Input: part model. Units: mm. Frame: model coordinates. Round coordinates to 2 decimals unless told otherwise and drop trailing zeros. Loops run counter-clockwise (first coordinate to the right, second up) from the corner with the lowest first, then second, coordinate; pieces in that order, holes last. Notation, with made-up numbers: (-11, 30.25) -> (25, 30.25) arc R19 ccw to (25, 51.25) -> close; hole circle Ø2 at (39.5, -36). An arc over 180 degrees is marked (long way). Answer in a Markdown table with one row per item. Add a question column.
Q1. Pin query (flat end, axial travel): pin 1 (2.5 mm diameter, centred on y = 2.5, z = 40.5, fed in from +X); pin 2 (1 mm diameter, centred on x = 11.5, y = 4, fed in from +Z); pin 3 (1 mm diameter, centred on x = -21, y = 4, fed in from +Z). Return the tip coordinate at first contact, or that it passes through.
Q2. Section C-C, the plane z = -30. Output: boundary loops of the cut face in (x, y).
Q3. Section A-A, the plane z = -63. Output: boundary loops of the cut face in (x, y).
Q4. Section B-B, the plane x = 40.5. Output: boundary loops of the cut face in (y, z).
Q5. Section D-D, the plane y = 1.2. Give the number of separate pieces and of enclosed holes in the cut face, and give its area (3 significant figures).
Q6. Ray query, L1, parallel to X at y = 4, z = -2; L2, parallel to Z at x = 66, y = 1.6; L3, parallel to Z at x = -39, y = 0.5. Return the intervals inside material, ascending. Write a range as from..to.
```python
from build123d import *

# Parameters (mm, degrees)
SKETCH1_R                = 95.25
SKETCH1_R_2              = 88.9
BOSS_EXTRUDE1_DEPTH      = 4.699
BOSS_EXTRUDE2_DEPTH      = 4.699
SKETCH3_R                = 12.7
BOSS_EXTRUDE3_DEPTH      = 4.699
BOSS_EXTRUDE4_DEPTH      = 4.699
FILLET1_R                = 3.175
CIRPATTERN1_COUNT        = 3
FILLET1_OF_CIRPATTERN1_R = 3.175
FILLET2_R                = 1.5875


with BuildPart() as part:
    # Sketch1 → Boss-Extrude1 (new body)
    with BuildSketch(Plane(origin=(0, 0, 0), x_dir=(1, 0, 0), z_dir=(0, 1, 0))):
        with Locations(Location((0, 0, 0), (0, 0, 270))):
            Circle(SKETCH1_R)
        with Locations(Location((0, 0, 0), (0, 0, 270))):
            Circle(SKETCH1_R_2, mode=Mode.SUBTRACT)
    extrude(amount=BOSS_EXTRUDE1_DEPTH)

    # Sketch2 → Boss-Extrude2 (add)
    with BuildSketch(Plane.XZ):
        with BuildLine():
            ThreePointArc((14.09030245, 107.026472785), (0, 107.95), (-14.09030245, 107.026472785))
            Line((-14.09030245, 107.026472785), (-12.432619809, 94.435123046))
            ThreePointArc((-12.432619809, 94.435123046), (0, 95.25), (12.432619809, 94.435123046))
            Line((12.432619809, 94.435123046), (14.09030245, 107.026472785))
        make_face()
        with BuildLine():
            Line((-15.09408047, -74.690084581), (-17.609760548, -87.138432012))
            ThreePointArc((-17.609760548, -87.138432012), (0, -88.9), (17.609760548, -87.138432012))
            Line((17.609760548, -87.138432012), (15.09408047, -74.690084581))
            ThreePointArc((15.09408047, -74.690084581), (0, -76.2), (-15.09408047, -74.690084581))
        make_face()
    extrude(amount=-BOSS_EXTRUDE2_DEPTH)



with BuildPart() as body_2:
    # Sketch3 → Boss-Extrude3 (new body)
    with BuildSketch(Plane.XZ):
        with Locations(Location((0, 0, 0), (0, 0, 270))):
            Circle(SKETCH3_R)
        Polygon((0, 5.499261314), (-4.7625, 2.749630657), (-4.7625, -2.749630657), (0, -5.499261314), (4.7625, -2.749630657), (4.7625, 2.749630657), align=None, mode=Mode.SUBTRACT)
    extrude(amount=-BOSS_EXTRUDE3_DEPTH)


with BuildPart() as part_1:
    add(part.part)

    add(body_2.part)  # Boss-Extrude4 merges body 2
    # Sketch4 → Boss-Extrude4 (add)
    with BuildSketch(Plane(origin=(0, 0, 0), x_dir=(-1, 0, 0), z_dir=(0, -1, 0))):
        with BuildLine():
            Line((3.175, -88.843285481), (3.175, -12.296722124))
            ThreePointArc((3.175, -12.296722124), (0, -12.7), (-3.175, -12.296722124))
            Line((-3.175, -12.296722124), (-3.175, -88.843285481))
            ThreePointArc((-3.175, -88.843285481), (0, -88.9), (3.175, -88.843285481))
        make_face()
    boss_extrude4 = extrude(amount=-BOSS_EXTRUDE4_DEPTH)

    # Fillet1
    fillet1_edges = [part_1.edges().sort_by_distance(p)[0] for p in [
        (-3.175, 2.3495, 12.296722124),
        (3.175, 2.3495, 12.296722124),
        (3.175, 2.3495, 88.843285481),
        (-3.175, 2.3495, 88.843285481),
    ]]
    fillet(fillet1_edges, radius=FILLET1_R)

    # CirPattern1: Boss-Extrude4 ×3 about axis
    cirpattern1_axis = Axis((0, 0, 0), (0, 1, 0))
    for i in range(1, CIRPATTERN1_COUNT):
        add(boss_extrude4.rotate(cirpattern1_axis, i * 360 / CIRPATTERN1_COUNT))

    # Fillet1 of CirPattern1
    fillet1_of_cirpattern1_edges = [part_1.edges().sort_by_distance(p)[0] for p in [
        (12.236773743, 2.3495, -3.398730405),
        (9.061773743, 2.3495, -8.897991719),
        (75.353042182, 2.3495, -47.171273397),
        (78.528042182, 2.3495, -41.672012083),
        (-9.061773743, 2.3495, -8.897991719),
        (-12.236773743, 2.3495, -3.398730405),
        (-78.528042182, 2.3495, -41.672012083),
        (-75.353042182, 2.3495, -47.171273397),
    ]]
    fillet(fillet1_of_cirpattern1_edges, radius=FILLET1_OF_CIRPATTERN1_R)

    # Fillet2
    fillet2_edges = [part_1.edges().sort_by_distance(p)[0] for p in [
        (-15.09408047, 2.3495, -74.690084581),
        (15.09408047, 2.3495, -74.690084581),
        (17.609760548, 2.3495, -87.138432012),
        (-17.609760548, 2.3495, -87.138432012),
        (-12.432619809, 2.3495, 94.435123046),
        (12.432619809, 2.3495, 94.435123046),
    ]]
    fillet(fillet2_edges, radius=FILLET2_R)


solid = part_1.part
```
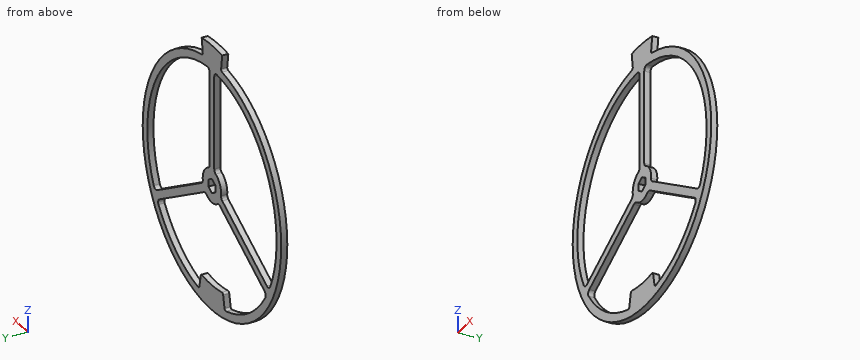
Answer block:
| question | item | result |
|---|---|---|
| 1 | pin 1 | x = 86.79 |
| 1 | pin 2 | z = 107.39 |
| 1 | pin 3 | z = 93.02 |
| 2 | outline | (-90.4, 0) -> (-83.69, 0) -> (-83.69, 4.7) -> (-90.4, 4.7) -> close; (-58.31, 0) -> (-45.61, 0) -> (-45.61, 4.7) -> (-58.31, 4.7) -> close; (45.61, 0) -> (58.31, 0) -> (58.31, 4.7) -> (45.61, 4.7) -> close; (83.69, 0) -> (90.4, 0) -> (90.4, 4.7) -> (83.69, 4.7) -> close |
| 3 | outline | (-71.44, 0) -> (-62.72, 0) -> (-62.72, 4.7) -> (-71.44, 4.7) -> close; (62.72, 0) -> (71.44, 0) -> (71.44, 4.7) -> (62.72, 4.7) -> close |
| 4 | outline | (0, -86.21) -> (4.7, -86.21) -> (4.7, -79.14) -> (0, -79.14) -> close; (0, -27.05) -> (4.7, -27.05) -> (4.7, -19.72) -> (0, -19.72) -> close; (0, 79.14) -> (4.7, 79.14) -> (4.7, 86.21) -> (0, 86.21) -> close |
| 5 | separate pieces | 1 |
| 5 | enclosed holes | 4 |
| 5 | area | 6,330 mm^2 |
| 6 | L1 | -95.23..-88.88, -12.61..-4.76, 4.76..12.61, 88.88..95.23 |
| 6 | L2 | -68.68..-59.56, -41.77..-34.44, 59.56..68.68 |
| 6 | L3 | -86.9..-79.89, -26.18..-18.85, 79.89..86.9 |
